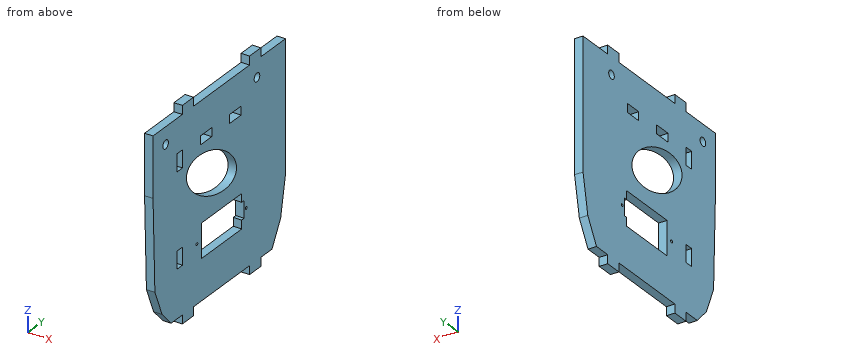
from build123d import *

# Parameters (mm, degrees)
SKETCH1_W                            = 71.755
SKETCH1_H                            = 57.15
MAIN_BODY_DEPTH                      = 3.175
SKETCH2_W                            = 3.2258
SKETCH2_H                            = 6.35
TABS_FRONT_DEPTH                     = 3.175
SKETCH3_R                            = 0.508
CUT_FOR_EAR_MOTOR_DEPTH              = 4.175
SKETCH4_W                            = 3.2258
SKETCH4_H                            = 6.477
SKETCH4_W_2                          = 6.477
SKETCH4_H_2                          = 3.2258
CUT_FOR_TABS_DEPTH                   = 4.175
BOSS_EXTRUDE1_DEPTH                  = 3.175
SKETCH6_R                            = 1.5875
CUT_FOR_FACE_PLATE_MOUNT_SCREW_DEPTH = 4.175
SKETCH7_RX                           = 15.24
SKETCH7_RY                           = 7.62
ELLIPSE_CUT_DEPTH                    = 4.175


with BuildPart() as part:
    # Sketch1 → main body (new body)
    with BuildSketch(Plane(origin=(0, 0, 0), x_dir=(0, 0, -1), z_dir=(1, 0, 0))):
        Rectangle(SKETCH1_W, SKETCH1_H)
    extrude(amount=MAIN_BODY_DEPTH)

    # Sketch2 → tabs front (add)
    with BuildSketch(Plane.ZY):
        with Locations((37.4904, 19.05)):
            Rectangle(SKETCH2_W, SKETCH2_H)
        with Locations((37.4904, -19.05)):
            Rectangle(SKETCH2_W, SKETCH2_H)
    tabs_front = extrude(amount=-TABS_FRONT_DEPTH)

    # mirror of tabs (back): tabs front across plane
    add(tabs_front.mirror(Plane.XY))

    # Sketch3 → cut for ear motor (cut, through all)
    with BuildSketch(Plane.ZY):
        with Locations((-14.356162211, 13.97)):
            Circle(SKETCH3_R)
        with Locations((-14.356162211, -13.97)):
            Circle(SKETCH3_R)
        Polygon((-20.706162211, -11.43), (-8.006162211, -11.43), (-8.006162211, 11.43), (-11.181162211, 11.43), (-11.181162211, 12.827), (-17.531162211, 12.827), (-17.531162211, 11.43), (-20.706162211, 11.43), align=None)
    extrude(amount=-CUT_FOR_EAR_MOTOR_DEPTH, mode=Mode.SUBTRACT)

    # Sketch4 → cut for tabs (cut, through all)
    with BuildSketch(Plane.ZY):
        with Locations((21.8186, 7.8613)):
            Rectangle(SKETCH4_W, SKETCH4_H)
        with Locations((21.8186, -8.7757)):
            Rectangle(SKETCH4_W, SKETCH4_H)
        with Locations((19.939, -23.7871)):
            Rectangle(SKETCH4_W_2, SKETCH4_H_2)
        with Locations((-14.859, -23.7871)):
            Rectangle(SKETCH4_W_2, SKETCH4_H_2)
    extrude(amount=-CUT_FOR_TABS_DEPTH, mode=Mode.SUBTRACT)

    # Sketch5 → Boss-Extrude1 (add)
    with BuildSketch(Plane.ZY):
        Polygon((-35.8775, -28.575), (35.8775, -28.575), (35.8775, -38.846719594), (13.523283037, -38.846719594), (-20.528592985, -37.801776478), (-30.363311769, -33.710859797), align=None)
        Polygon((-12.787335482, 36.195), (-27.046355521, 33.492436966), (-35.8775, 28.575), (35.8775, 28.575), (35.8775, 36.195), (26.200162008, 36.195), align=None)
    extrude(amount=-BOSS_EXTRUDE1_DEPTH)

    # Sketch6 → cut for face plate mount screw (cut, through all)
    with BuildSketch(Plane.ZY):
        with Locations((29.5275, 20.066)):
            Circle(SKETCH6_R)
        with Locations((29.5275, -31.734719594)):
            Circle(SKETCH6_R)
    extrude(amount=-CUT_FOR_FACE_PLATE_MOUNT_SCREW_DEPTH, mode=Mode.SUBTRACT)

    # Sketch7 → ellipse cut (cut, through all)
    with BuildSketch(Plane.ZY):
        with Locations(Location((7.3025, -5.715), (0, 0, -65))):
            Ellipse(SKETCH7_RX, SKETCH7_RY)
    extrude(amount=-ELLIPSE_CUT_DEPTH, mode=Mode.SUBTRACT)


solid = part.part
Could you check a few things on this model? Use its own coordinates, in mm. Give positions to 0.01 mm unless a question says otherwise; leave off trailing zeros. Order: outer loops, then holes, each group sorted by start corner. A loop starts at its lowest first (then second) coordinate and runs counter-clockwise, first axis right, second up.
1. Suppose I cut it at A-A (y = -10). Give the number of separate pieces and of enclosed holes in the cut face, plus the area to 3 significant figures.
2. Will these pins go through, and if not, where does the flat tip stop? P1, Ø1, axis at x = 1, y = -24.5, coming from the +Z side; P2, Ø1, axis at y = 25, z = 3, coming from the -X side; P3, Ø1.6, axis at x = 2.5, y = -26.5, coming from the -Z side; P4, Ø1.6, axis at x = 1.5, z = -37, coming from the +Y side (3 decimals).
3. Suppose I cut it at C-C (y = 29.5). List the corners of the cut face in (x, z) for me (1 decimal).
4. I need wall thicknesses on L1, parallel to Z at x = 0.95, y = 9; L2, parallel to Y at x = 1.2, z = 29 (3 decimals); L3, parallel to Z at x = 0.2, y = -23.5. Which ranges of each line are inside material? Lowest first, please.
Solved:
1. separate pieces: 4
1. enclosed holes: 0
1. area: 128 mm2
2. P1: stops at z = 35.88
2. P2: stops at x = 0
2. P3: stops at z = -35.88
2. P4: stops at y = 22.225
3. outline: (0, -34.2) - (3.2, -34.2) - (3.2, 35.9) - (0, 35.9) - close
4. L1: z = -35.88 to -20.71, -8.01 to 20.21, 23.43 to 35.88
4. L2: y = -38.847 to -33.232, -30.237 to 18.569, 21.563 to 36.195
4. L3: z = -35.88 to -18.1, -11.62 to 16.7, 23.18 to 35.88
